Geometry: see drawing. Coordinates: mm, zero at the bounding-box minimum. A direction names the side the tool comes from. Round coordinates to 2 decimals unless told otherwise and drop trailing zeros. Order: outer loops, then holes, each group sorted by start corner. A loop starts at its lowest first (then second) coordinate and runs counter-clockwise, first axis right, second up. Notation, with made-up numbers: (-24.75, 76) -> (-1.75, 76) arc R9 ccw to (-1.75, 89) -> close; hole circle Ø1 at (42.5, 86). An arc over 180 degrees is marked (long way). Use a Markdown table: item, result.
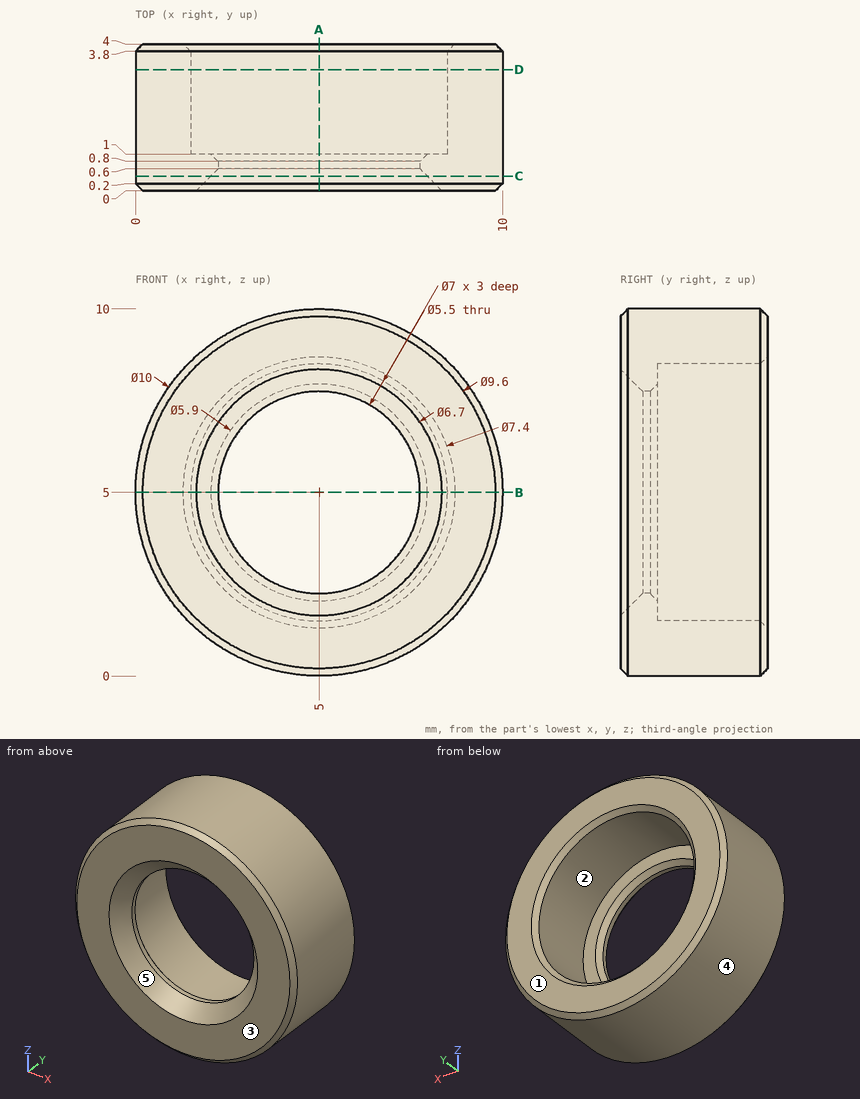
1) Contact query for flat-ended pins moving along their axis: P1, Ø1, axis at y = 2.5, z = 4, coming from the +X side; P2, Ø2, axis at x = 2.5, y = 3.5, coming from the +Z side. Output: stop coordinate, or through.
Answer key:
| item | result |
|---|---|
| P1 | stops at x = 9.97 |
| P2 | stops at z = 9.77 |
2) Ray query, probe 1 along Z at (x, y) = (5, 0.7); probe 2 along Z at (x, y) = (5, 3.2). Return the intervals inside material, ascending.
Answer key:
| item | result |
|---|---|
| probe 1 | z = 0 to 2.25, 7.75 to 10 |
| probe 2 | z = 0 to 1.5, 8.5 to 10 |
3) Cut plane C-C on y = 0.4. Return loops of the section in (x, z).
Answer key:
| item | result |
|---|---|
| outline | circle Ø10 at (5, 5); hole circle Ø5.9 at (5, 5) |
4) Cut plane D-D on y = 3.3. Return loops of the section in (x, z).
Answer key:
| item | result |
|---|---|
| outline | circle Ø10 at (5, 5); hole circle Ø7 at (5, 5) |
5) Cut plane A-A on x = 5. Return loops of the section in (y, z).
Answer key:
| item | result |
|---|---|
| outline | (0, 0.2) -> (0.2, 0) -> (3.8, 0) -> (4, 0.2) -> (4, 1.3) -> (3.8, 1.5) -> (1, 1.5) -> (1, 2.05) -> (0.8, 2.25) -> (0.6, 2.25) -> (0, 1.65) -> close; (0, 8.35) -> (0.6, 7.75) -> (0.8, 7.75) -> (1, 7.95) -> (1, 8.5) -> (3.8, 8.5) -> (4, 8.7) -> (4, 9.8) -> (3.8, 10) -> (0.2, 10) -> (0, 9.8) -> close |
6) Cut plane B-B on z = 5. Return loops of the section in (x, y), and give its area (3 significant figures).
Answer key:
| item | result |
|---|---|
| outline | (0, 0.2) -> (0.2, 0) -> (1.65, 0) -> (2.25, 0.6) -> (2.25, 0.8) -> (2.05, 1) -> (1.5, 1) -> (1.5, 3.8) -> (1.3, 4) -> (0.2, 4) -> (0, 3.8) -> close; (7.75, 0.6) -> (8.35, 0) -> (9.8, 0) -> (10, 0.2) -> (10, 3.8) -> (9.8, 4) -> (8.7, 4) -> (8.5, 3.8) -> (8.5, 1) -> (7.95, 1) -> (7.75, 0.8) -> close |
| area | 13.0 mm^2 |
7) Set-up query: the marked faces 1 and 2. Return all of +Z, -Z, +X, -X, +Y, -Y with unobstructed straight access to the full face (end or side cutting, diameter ignored); none if empty.
Answer key:
| item | result |
|---|---|
| face 1 | +Z, -Z, +X, -X, +Y |
| face 2 | +Y |
8) Draft query along Z for the marked faces 3, 4 and 5. Return one class per face: released by +Z, released by -Z, zero draft, split by the parting line, or undercut.
Answer key:
| item | result |
|---|---|
| face 3 | zero draft |
| face 4 | split by the parting line |
| face 5 | undercut |
